```python
from build123d import *

# Parameters (mm, degrees)
SKETCH1_W           = 103.6
SKETCH1_H           = 63.3
BOSS_EXTRUDE1_DEPTH = 0.4
SKETCH2_W           = 14
SKETCH2_H           = 16
CUT_EXTRUDE1_DEPTH  = 61.705209826
CUT_EXTRUDE2_DEPTH  = 61.705209826
LPATTERN1_COUNT     = 2
LPATTERN1_PITCH     = 15
LPATTERN1_COL_COUNT = 2
LPATTERN1_COL_PITCH = 15


with BuildPart() as part:
    # Sketch1 → Boss-Extrude1 (new body)
    with BuildSketch(Plane(origin=(0, 0, 0), x_dir=(1, 0, 0), z_dir=(0, 1, 0))):
        Rectangle(SKETCH1_W, SKETCH1_H)
    extrude(amount=-BOSS_EXTRUDE1_DEPTH)

    # Sketch2 → Cut-Extrude1 (cut, through all)
    with BuildSketch(Plane(origin=(0, 0, 0), x_dir=(1, 0, 0), z_dir=(0, 1, 0))):
        with Locations((42.5, 13.25)):
            Rectangle(SKETCH2_W, SKETCH2_H)
    extrude(amount=-CUT_EXTRUDE1_DEPTH, mode=Mode.SUBTRACT)

    # Sketch3 → Cut-Extrude2 (cut, through all)
    with BuildSketch(Plane(origin=(0, 0, 0), x_dir=(1, 0, 0), z_dir=(0, 1, 0))):
        with BuildLine():
            Line((0.707106781, -8.921572875), (2.828427125, -11.042893219))
            ThreePointArc((2.828427125, -11.042893219), (2.828427125, -14.578427125), (-0.707106781, -14.578427125))
            Line((-0.707106781, -14.578427125), (-2.828427125, -12.457106781))
            ThreePointArc((-2.828427125, -12.457106781), (-2.828427125, -8.921572875), (0.707106781, -8.921572875))
        make_face()
    cut_extrude2 = extrude(amount=-CUT_EXTRUDE2_DEPTH, mode=Mode.SUBTRACT)

    # LPattern1: Cut-Extrude2 ×2
    with Locations(*[(i * LPATTERN1_PITCH, 0, 0) for i in range(1, LPATTERN1_COUNT)]):
        add(cut_extrude2, mode=Mode.SUBTRACT)

    # LPattern1 col: Cut-Extrude2 ×2
    with Locations(*[(-i * LPATTERN1_COL_PITCH, 0, 0) for i in range(1, LPATTERN1_COL_COUNT)]):
        add(cut_extrude2, mode=Mode.SUBTRACT)


solid = part.part
```
Could you check a few things on this model? Use its own coordinates, in mm. A direction names the side the tool comes from. Round coordinates to 2 decimals unless told otherwise and drop trailing zeros. Loops run counter-clockwise (first coordinate to the right, second up) from the corner with the lowest first, then second, coordinate; pieces in that order, holes last. Notation, with made-up numbers: (33, 19.5) - (92, 19.5) arc R23 cw to (92, 56.5) - close; hole circle Ø9 at (73.5, 18). An arc over 180 degrees is marked (long way). Answer in a Markdown table with one row per item. Add a question column.
(1) If we mould it in two halves opening along Z, with no side actions, what happens to faces 1 (the face through (-17.867, -0.197, 8.961)), 2 (the face through (-1, 0, 0))? For each: pulls with the +Z half, pulls with the -Z half, needs draft (parallel to the pull), parting line crosses it, or undercut.
(2) I need wall thicknesses on line 1 along Z through (x, y) = (42, -0.3); line 2 along X through (y, z) = (-0.1, 14.5); line 3 along X through (y, z) = (-0.3, -9). Which ranges of each line are inside material? Lowest first, please.
(3) If we section it at C-C (z = -7.5): Please give me the cut outline in (x, y), plus the area to 3 significant figures.
(4) If we section it at A-A (y = -0.25): Please give me the cut outline in (x, z), plus the area to 3 significant figures.
(5) For faces 3 (the face through (-1, -0.4, 0)), 4 (the face through (-13.247, -0.197, 9.967)), which set-ups out of +Z, -Z, +X, -X, +Y, -Y let a thin tool reach every point of the face, with its end or its side?
(6) If we section it at B-B (x = 45.5): Please give me the cut outline in (y, z), plus the area to 3 significant figures.
Model answer:
| question | item | result |
|---|---|---|
| 1 | face 1 | undercut |
| 1 | face 2 | needs draft |
| 2 | line 1 | z = -31.65 to -21.25, -5.25 to 31.65 |
| 2 | line 2 | x = -51.8 to -15.79, -12.1 to -0.79, 2.9 to 14.21, 17.9 to 51.8 |
| 2 | line 3 | x = -51.8 to 35.5, 49.5 to 51.8 |
| 3 | outline | (-51.8, -0.4) - (35.5, -0.4) - (35.5, 0) - (-51.8, 0) - close; (49.5, -0.4) - (51.8, -0.4) - (51.8, 0) - (49.5, 0) - close |
| 3 | area | 35.8 mm² |
| 4 | outline | (-51.8, -31.65) - (51.8, -31.65) - (51.8, 31.65) - (-51.8, 31.65) - close; hole (-17.83, 12.46) arc R2.5 ccw to (-14.29, 8.92) - (-12.17, 11.04) arc R2.5 ccw to (-15.71, 14.58) - close; hole (-2.83, 12.46) arc R2.5 ccw to (0.71, 8.92) - (2.83, 11.04) arc R2.5 ccw to (-0.71, 14.58) - close; hole (12.17, 12.46) arc R2.5 ccw to (15.71, 8.92) - (17.83, 11.04) arc R2.5 ccw to (14.29, 14.58) - close; hole (35.5, -21.25) - (49.5, -21.25) - (49.5, -5.25) - (35.5, -5.25) - close |
| 4 | area | 6,230 mm² |
| 5 | face 3 | +Z, -Z, +X, -X, -Y |
| 5 | face 4 | +Y, -Y |
| 6 | outline | (-0.4, -31.65) - (0, -31.65) - (0, -21.25) - (-0.4, -21.25) - close; (-0.4, -5.25) - (0, -5.25) - (0, 31.65) - (-0.4, 31.65) - close |
| 6 | area | 18.9 mm² |
